from build123d import *

# Parameters (mm, degrees)
F0_W     = 15
F0_H     = 15
F1_DEPTH = 30
F2_W     = 15
F2_H     = 10
F3_DEPTH = 80
F4_R     = 4.99999
F5_W     = 10
F5_H     = 10
F6_DEPTH = 20


# Not quite as in the source:
# - a fillet or chamfer is up to 0.001 mm smaller than in the source, because OpenCascade refuses the exact size


with BuildPart() as f1:
    # F0 (on Top) → F1 (new body)
    with BuildSketch(Plane.XY):
        Rectangle(F0_W, F0_H)
    extrude(amount=F1_DEPTH)

    # F2 (on face) → F3 (join)
    with BuildSketch(Plane.XZ.offset(7.5)):
        with Locations((0, 25)):
            Rectangle(F2_W, F2_H)
    extrude(amount=F3_DEPTH)

    # F4 (radius 5 in the source; OpenCascade refuses exactly that, so slightly less here)
    f4_edges = [f1.edges().sort_by_distance(p)[0] for p in [
        (7.5, -40, 30),
        (-7.5, -40, 30),
        (7.5, -47.5, 20),
        (-7.5, -47.5, 20),
    ]]
    fillet(f4_edges, radius=F4_R)

    # F5 (on face) → F6 (cut)
    with BuildSketch(Plane(origin=(0, 0, 0), x_dir=(1, 0, 0), z_dir=(0, 0, -1))):
        Rectangle(F5_W, F5_H)
    extrude(amount=-F6_DEPTH, mode=Mode.SUBTRACT)


solid = f1.part
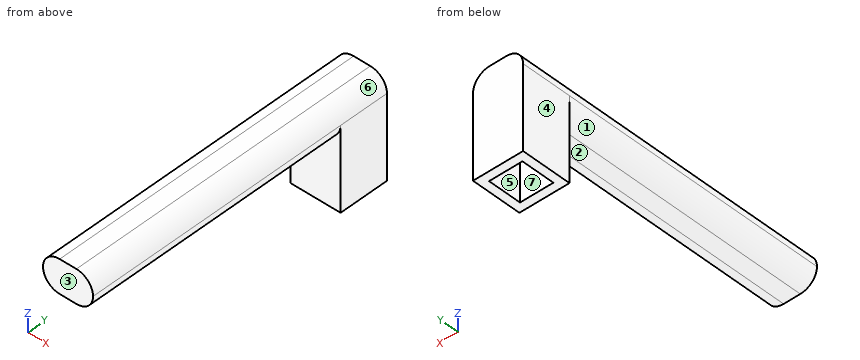
Check sheet for the modelled part. Datum: model origin and axes. Units: mm. Face numbers are marked on the shaded views. A direction names the side the tool comes from. Round coordinates to 2 decimals unless told otherwise and drop trailing zeros. Order: outer loops, then holes, each group sorted by start corner. A loop starts at its lowest first (then second) coordinate and runs counter-clockwise, first axis right, second up.
Q1. Cross-section at B-B, the plane x = -1.5. Enter the section's corners in (y, z).
Filled sheet:
outline: (-87.5, 20) - (-7.5, 20) - (-7.5, 0) - (-5, 0) - (-5, 20) - (5, 20) - (5, 0) - (7.5, 0) - (7.5, 30) - (-87.5, 30) - close
Q2. Cross-section at D-D, the plane z = 23.25. Enter the section's corners in (x, y), plus the area to 3 significant figures.
Filled sheet:
outline: (-7.5, -7.5) - (-7.18, -7.5) - (-7.18, -87.5) - (7.18, -87.5) - (7.18, -7.5) - (7.5, -7.5) - (7.5, 7.5) - (-7.5, 7.5) - close
area: 1,370 mm2
Q3. Set-up check for the marked faces 1, 2 and 3: record each of +Z, -Z, +X, -X, +Y, -Y from which the full face is reachable in a straight line by a thin tool's end or side.
Filled sheet:
face 1: -Z, -X, -Y
face 2: -Z, +X, -X, -Y
face 3: +Z, -Z, +X, -X, -Y
Q4. Draft check along X on the marked faces 4, 5, 6 and 7. Enter one of: pulls with the +X half, pulls with the -X half, needs draft (parallel to the pull), parting line crosses it, or undercut.
Filled sheet:
face 4: pulls with the -X half
face 5: undercut
face 6: pulls with the +X half
face 7: undercut
Q5. Scan lines: L1, parallel to Y at x = -0.75, z = 14.5; L2, parallel to Z at x = -2.25, y = -28; L3, parallel to Y at x = 6.5, z = 9. Record each from-to range of solid material in increasing order.
Filled sheet:
L1: y = -7.5 to -5, 5 to 7.5
L2: z = 20 to 30
L3: y = -7.5 to 7.5
Q6. Depth check by flat-ended pin: P1, Ø3, axis at x = -4.5, y = -61, coming from the +Z side; P2, Ø4, axis at x = 0.5, y = -57.5, coming from the -Z side; P3, Ø12, axis at y = -18.5, z = 15.5, coming from the -X side. Enter the tip coordinate at first touch or a pass-through.
Filled sheet:
P1: stops at z = 29.97
P2: stops at z = 20
P3: stops at x = -6.07
Q7. Cross-section at A-A, the plane z = 4. Enter the section's corners in (x, y).
Filled sheet:
outline: (-7.5, -7.5) - (7.5, -7.5) - (7.5, 7.5) - (-7.5, 7.5) - close; hole (-5, -5) - (5, -5) - (5, 5) - (-5, 5) - close
